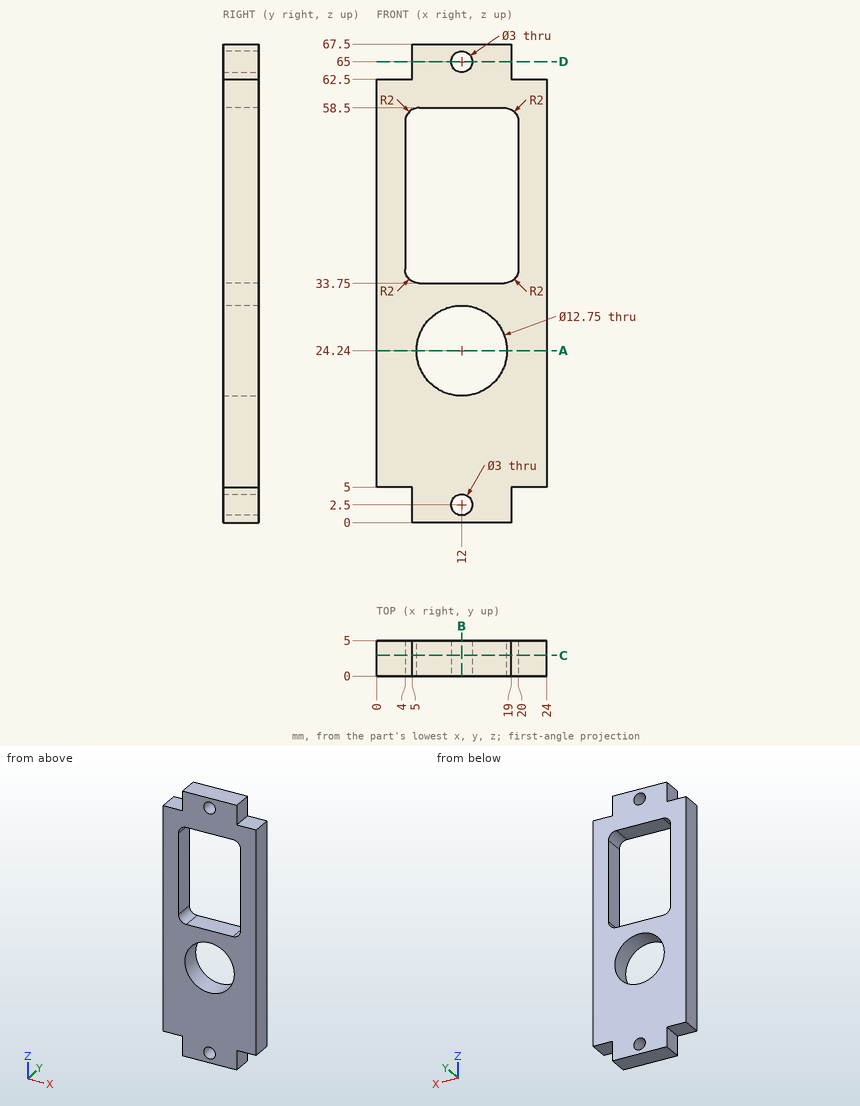
Drawing for the job (mm, zero at the part's lowest x, y, z). Round coordinates to 2 decimals unless told otherwise and drop trailing zeros. Order: outer loops, then holes, each group sorted by start corner. A loop starts at its lowest first (then second) coordinate and runs counter-clockwise, first axis right, second up. Notation, with made-up numbers: (15.5, 33.25) -> (38.5, 33.25) arc R32 ccw to (38.5, 62.25) -> close; hole circle Ø11 at (-14, -31). An arc over 180 degrees is marked (long way). Put each result on its own line as item: value.
Q1. Band-saw the part on B-B (x = 12). Give the cut face in (y, z) (3 decimals).
From the geometry:
outline: (0, 0) -> (5, 0) -> (5, 1) -> (0, 1) -> close; (0, 4) -> (5, 4) -> (5, 17.865) -> (0, 17.865) -> close; (0, 30.615) -> (5, 30.615) -> (5, 33.75) -> (0, 33.75) -> close; (0, 58.5) -> (5, 58.5) -> (5, 63.5) -> (0, 63.5) -> close; (0, 66.5) -> (5, 66.5) -> (5, 67.5) -> (0, 67.5) -> close
Q2. Pin check, flat tips, straight feed: pin 1 Ø11.5 at (x, z) = (12, 24.24) entering from +Y; pin 2 Ø1.5 at (y, z) = (2, 3.5) entering from +X; pin 3 Ø1.5 at (y, z) = (3.5, 66) entering from -X; pin 4 Ø1.5 at (x, y) = (3.5, 3) entering from -Z. Stop position of each tip, or through.
From the geometry:
pin 1: passes through
pin 2: stops at x = 19
pin 3: stops at x = 5
pin 4: stops at z = 5
Q3. Band-saw the part on A-A (z = 24.24). Give the cut face in (x, y) (3 decimals), and give its area (4 significant figures).
From the geometry:
outline: (0, 0) -> (5.625, 0) -> (5.625, 5) -> (0, 5) -> close; (18.375, 0) -> (24, 0) -> (24, 5) -> (18.375, 5) -> close
area: 56.25 mm2
Q4. Band-saw the part on C-C (y = 2.9). Give the cut face in (x, z) (3 decimals).
From the geometry:
outline: (0, 5) -> (5, 5) -> (5, 0) -> (19, 0) -> (19, 5) -> (24, 5) -> (24, 62.5) -> (19, 62.5) -> (19, 67.5) -> (5, 67.5) -> (5, 62.5) -> (0, 62.5) -> close; hole (4, 35.75) arc R2 ccw to (6, 33.75) -> (18, 33.75) arc R2 ccw to (20, 35.75) -> (20, 56.5) arc R2 ccw to (18, 58.5) -> (6, 58.5) arc R2 ccw to (4, 56.5) -> close; hole circle Ø12.75 at (12, 24.24); hole circle Ø3 at (12, 2.5); hole circle Ø3 at (12, 65)
Q5. Band-saw the part on D-D (z = 65). Give the cut face in (x, y), and give its area (3 significant figures).
From the geometry:
outline: (5, 0) -> (10.5, 0) -> (10.5, 5) -> (5, 5) -> close; (13.5, 0) -> (19, 0) -> (19, 5) -> (13.5, 5) -> close
area: 55.0 mm2
Q6. Wall check: line 1 (X direction, y = 1.3, z = 40); line 2 (Z direction, x = 10, y = 4.15); line 3 (X direction, y = 2.85, z = 24.5). Give the ranges that are in metal, low to high. Write a range as [from, to].
From the geometry:
line 1: x = [0, 4], [20, 24]
line 2: z = [0, 18.19], [30.29, 33.75], [58.5, 67.5]
line 3: x = [0, 5.63], [18.37, 24]
